Input: part model. Units: mm. Frame: model coordinates. A direction names the side the tool comes from. Round coordinates to 2 decimals unless told otherwise and drop trailing zeros. Order: outer loops, then holes, each group sorted by start corner. A loop starts at its lowest first (then second) coordinate and runs counter-clockwise, first axis right, second up. Notation, with made-up numbers: (47, -25.5) -> (89, -25.5) arc R23 cw to (89, -16.5) -> close; hole circle Ø6 at (49, -10.75). An arc over 180 degrees is marked (long way). Use a Markdown table: item, result.
Autodesk Inventor part; units mm, degrees
ref_plane "YZ Plane" through (0, 0, 0) normal (1, 0, 0) x (0, 1, 0)
ref_plane "XZ Plane" through (0, 0, 0) normal (0, 1, 0) x (-1, 0, 0)
ref_plane "XY Plane" through (0, 0, 0) normal (0, 0, 1) x (1, 0, 0)
sketch "Sketch1" plane through (0, 0, 0) normal (0, 0, 1) x (1, 0, 0)
  line L0 (0, 0) -> (5, 0)
  line L1 (5, 0) -> (5, 95)
  line L2 (5, 95) -> (2.5, 95)
  line L3 (0, 92.4007) -> (0, 0)
  arc A0 (-2.5, 100) -> (2.5, 95) centre (2.5, 100) ccw
  arc A1 (-5.5, 100) -> (0, 92.4007) centre (2.5, 100) ccw
  line L4 (-5.5, 100) -> (-2.5, 100)
  point P0 (2.5, 0)
  dimension "d1" = 95
  dimension "d5" = 10
  dimension "d6" = 3
  dimension "d7" = 3
  dimension "d8" = 5
extrude "Extrusion1" add sketch "Sketch1" along normal blind 3
fillet "Fillet2" radius 1.5 2 edges at (-2.5, 100, 1.5) (-5.5, 100, 1.5)
sketch "Sketch3" plane through (0, 0, 3) normal (0, 0, 1) x (1, 0, 0)
  line L0 (0, 95.6699) -> (5, 92.9)
  line L1 (5, 92.9) -> (5, 95)
  line L2 (5, 95) -> (0, 95.6699)
  arc A0 (-2.365, 98.8462) -> (2.5, 95) centre (2.5, 100) ccw
  point P0 (0, 0)
  point P1 (0, 92.4007)
  dimension "d12" = 5
  dimension "d14" = 2.1
extrude "Extrusion2" cut sketch "Sketch3" against normal through all
properties part number "Moving Ramp Holder Shaft"
1) Cut plane C-C on x = 2.5. Return loops of the section in (y, z).
Answer key:
| item | result |
|---|---|
| outline | (0, 0) -> (94.28, 0) -> (94.28, 3) -> (0, 3) -> close |
2) Ray query, probe 1 along X at (y, z) = (42.5, 2.45); probe 2 along Y at (x, z) = (1.5, 1.9); probe 3 along Y at (x, z) = (-0.5, 0.4). Return the intervals inside material, ascending.
Answer key:
| item | result |
|---|---|
| probe 1 | x = 0 to 5 |
| probe 2 | y = 0 to 94.84 |
| probe 3 | y = 92.58 to 96 |
3) Cut plane B-B on y = 49. Return loops of the section in (x, z).
Answer key:
| item | result |
|---|---|
| outline | (0, 0) -> (5, 0) -> (5, 3) -> (0, 3) -> close |
4) Set-up query: faces 1 (the face through (0, 47, 1)), 2 (the face through (2, 0, 1)). Return all of +Z, -Z, +X, -X, +Y, -Y with unobstructed straight access to the full face (end or side cutting, diameter ignored); none if empty.
Answer key:
| item | result |
|---|---|
| face 1 | +Z, -Z, -X, -Y |
| face 2 | +Z, -Z, +X, -X, -Y |
5) Contact query for flat-ended pins moving along their axis: P1, Ø0.9, axis at y = 27.5, z = 1.5, coming from the -X side; P2, Ø1.5, axis at x = -2, z = 2.5, coming from the -Y side. Output: stop coordinate, or through.
Answer key:
| item | result |
|---|---|
| P1 | stops at x = 0 |
| P2 | stops at y = 92.93 |
